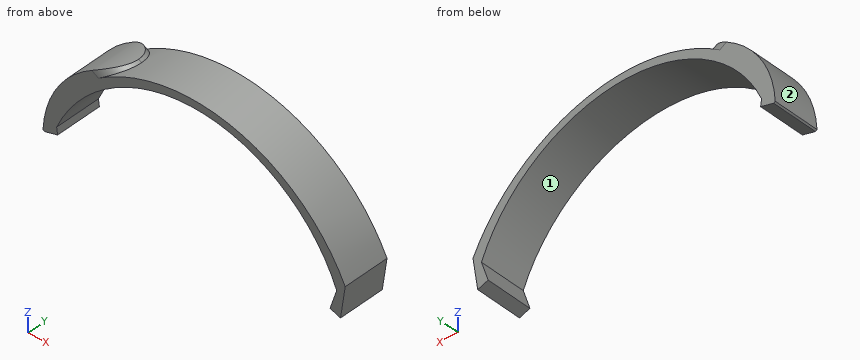
Autodesk Inventor part; units mm, degrees
ref_plane "YZ Plane" through (0, 0, 0) normal (1, 0, 0) x (0, 1, 0)
ref_plane "XY Plane" through (0, 0, 0) normal (0, 0, 1) x (1, 0, 0)
ref_plane "Work Plane1" through (0, -273.05, 0) normal (0, 1, 0) x (-1, 0, 0)
sketch "Sketch1" plane through (0, -273.05, 0) normal (0, 1, 0) x (-1, 0, 0)
  line L0 (28.2313, 0) -> (-81.8149, 0)
  point P0 (0, 0)
ref_plane "Work Plane2" through (-28.2313, -273.05, 0) normal (0, 0.9994, 0.0349) x (1, 0, 0)
sketch "Sketch2" plane through (-28.2313, -273.05, 0) normal (0, 0.9994, 0.0349) x (1, 0, 0)
  ellipse E0 centre (142.9444, 40.4167) end of major axis (127.2199, 83.6456) minor radius 0.5491 (135.3201, 59.9472) -> (144.2427, 35.2519) ccw
  ellipse E1 centre (145.4346, 41.3225) end of major axis (129.7101, 84.5514) minor radius 0.5491 (137.8103, 60.853) -> (146.7329, 36.1577) ccw
  line L0 (144.2427, 35.2519) -> (146.7329, 36.1577)
  ellipse E2 centre (-15.3961, 31.7454) end of major axis (-31.1205, -11.4836) minor radius 0.5491 (-17.0369, 25.6432) -> (-8.0746, 50.4278) ccw
  line L1 (-17.0369, 25.6432) -> (-19.5271, 26.549)
  ellipse E3 centre (-17.8862, 32.6512) end of major axis (-33.6107, -10.5778) minor radius 0.5491 (-19.5271, 26.549) -> (-10.5647, 51.3336) ccw
  line L2 (-19.5271, 32.4296) -> (-18.2659, 22.0654)
  arc A0 (-18.2659, 22.0654) -> (148.9119, 28.6146) centre (63.7007, 66.7506) ccw
  line L3 (148.9119, 28.6146) -> (145.6991, 46.4313)
  line L4 (145.6991, 46.4313) -> (139.9268, 44.3316)
  line L5 (139.9268, 44.3316) -> (144.0175, 33.0855)
  line L6 (-19.5271, 32.4296) -> (-12.1574, 30.5326)
  line L7 (-12.1574, 30.5326) -> (-12.6035, 26.6966)
  arc A1 (-12.6035, 26.6966) -> (144.0175, 33.0855) centre (64.3823, 62.3675) ccw
  line L8 (24.7417, -18.0874) -> (23.158, -19.0562)
  arc A2 (-20.3945, 31.8123) -> (23.158, -19.0562) centre (36.4902, 36.4371) ccw
  line L9 (-20.3945, 31.8123) -> (-19.5271, 32.4296)
  point P0 (28.2313, 9.5293)
  point P1 (-19.007, 27.8025)
  point P2 (140.8209, 44.6568)
  point P3 (-14.9879, 31.2612)
  point P4 (-17.0369, 25.6432)
  point P5 (-18.7784, 26.2767)
  point P6 (143.311, 45.5626)
  point P7 (-19.5271, 26.549)
  point P8 (-18.9903, 28.0182)
extrude "Extrusion1" add sketch "Sketch2" along normal blind 25.4
fillet "Fillet1" radius 12.7 2 edges at (-4.2815, -248.3136, 19.4469) (-4.2815, -273.6981, 18.5605)
properties part number "thigh_strap_05"
Can you work these out from the model? Positions are in its coordinate system, mm. Face numbers are marked on the shaded views. Coordinates: 2 decimals unless noted, no trailing zeros. Loops run counter-clockwise (first coordinate to the right, second up) from the corner with the lowest first, then second, coordinate; pieces in that order, holes last. Notation, with made-up numbers: (-26, -39.5) -> (33, -39.5) arc R12 ccw to (33, -32.5) -> close; hole circle Ø2 at (66.5, -13). An arc over 180 degrees is marked (long way). Answer as a JSON object with one key per item and string values.
1) Imagine slicing it at B-B (z = -39.5). Please give me the cut outline in (x, y).
Results:
{"outline": "(113.12, -246.26) -> (113.44, -271.67) -> (118.71, -271.67) -> (118.55, -246.26) -> close"}
2) For P1, Ø2, axis at y = -252.5, z = -26, coming from the -X side; P2, Ø3, axis at x = 23, z = 18, coming from the +Y side; P3, Ø3, axis at x = 45.5, y = -259.5, coming from the +Z side; P4, Ø5, axis at x = 78, y = -263, coming from the -Z side, each with a flat end and sliding along its axis, tell me the tip position at first contact or that it passes through.
Results:
{"P1": "stops at x = -48.14", "P2": "passes through", "P3": "stops at z = 26.71", "P4": "stops at z = 10.32"}
3) Imagine slicing it at A-A (x = 77). Please give me the cut outline in (y, z).
Results:
{"outline": "(-273.64, 16.85) -> (-273.47, 11.99) -> (-248.08, 12.88) -> (-248.25, 17.73) -> close"}
4) If I drill on line 1 (X direction, y = -254.75, z = -10); line 2 (X direction, y = -258.5, z = 2.5); line 3 (Z direction, x = 34, y = -259.5), over which ranges is the centre line in solid material (lowest first)?
Results:
{"line 1": "x = -42.65 to -31.1, 103.4 to 110.08", "line 2": "x = -33.94 to -19.14, 91.44 to 98.64", "line 3": "z = 22.94 to 27.08"}
5) Thinking about a two-plate mould opening in X: for the marked faces 1 and 2, which applies, pulls with the +X half, pulls with the -X half, needs draft (parallel to the pull), parting line crosses it, or undercut?
Results:
{"face 1": "undercut", "face 2": "pulls with the -X half"}
